Job drawing, mm, ordinate dimensions from the low corner. One solid piece. Coordinates: 2 decimals unless noted, no trailing zeros. Write each loop counter-clockwise with the first axis right and the second up, starting at its lowest first coordinate (ties: lowest second). Pieces come first, ordered by that corner, then holes. Notation, with made-up numbers: (-12, 26) -> (40, 26) arc R29 cw to (40, 52) -> close; hole circle Ø4 at (-24.75, 73.25). An arc over 180 degrees is marked (long way). Answer as a JSON object with one key per item and string values. Group by question number.
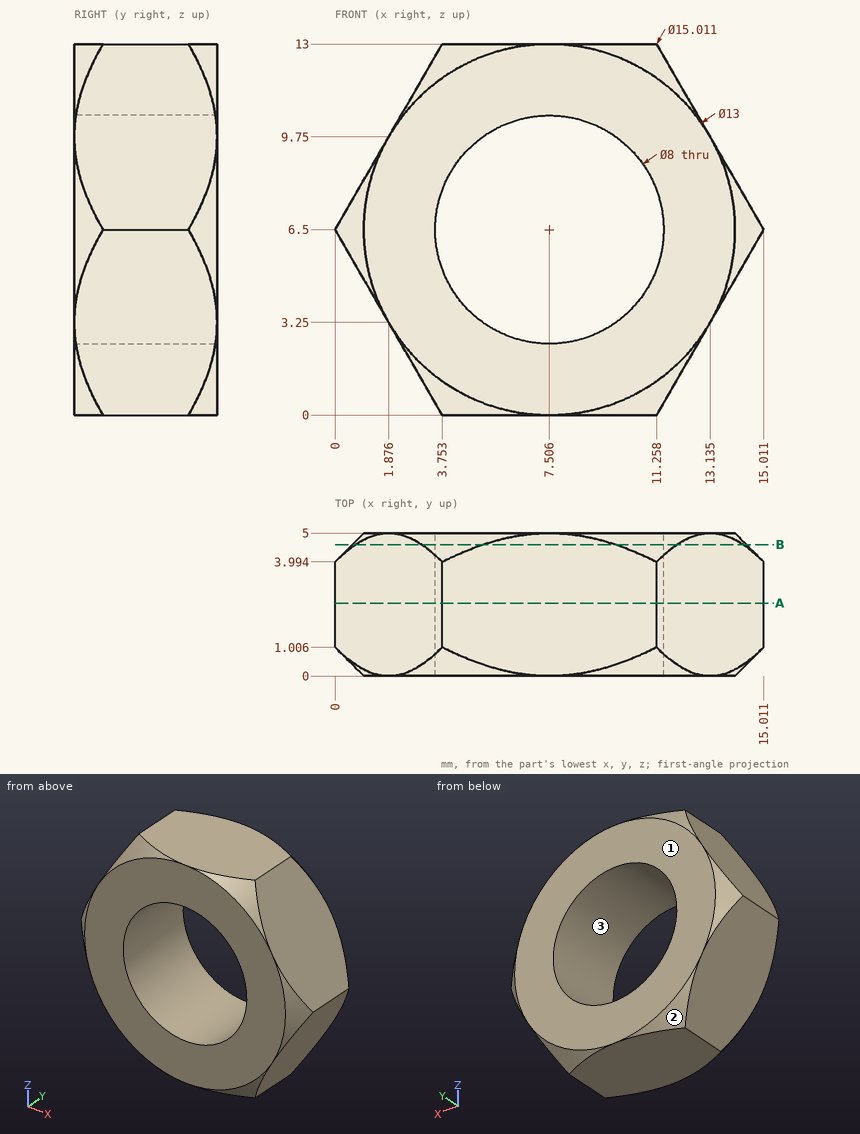
(1) Pin check, flat tip, straight feed: pin 1 (3 mm diameter, centred on y = 2, z = 3.5, fed in from -X) (1 decimal). Stop position of the tip, or through.
(2) Cut at A-A on y = 2.55. List the corners of the cut face in (x, z) (1 decimal).
(3) Pull direction X, two halves, no side cores. Call the marked faces 1, 2 and 3: released by +X, released by -X, zero draft, split by the parting line, or undercut.
(4) Wall check: probe 1 along Z at (x, y) = (6.25, 2.2); probe 2 along X at (y, z) = (1.5, 7.25) (1 decimal); probe 3 along Z at (x, y) = (7, 0.95). Give the ranges that are in metal, low to high.
(5) Cut at B-B on y = 4.6. List the corners of the cut face in (x, z) (1 decimal).
Results found:
{
 "1": {"pin 1": "stops at x = 0.9"},
 "2": {"outline": "(0, 6.5) -> (3.8, 0) -> (11.3, 0) -> (15, 6.5) -> (11.3, 13) -> (3.8, 13) -> close; hole circle Ø8 at (7.5, 6.5)"},
 "3": {"face 1": "zero draft", "face 2": "released by -X", "face 3": "undercut"},
 "4": {"probe 1": "z = 0 to 2.7, 10.3 to 13", "probe 2": "x = 0.4 to 3.6, 11.4 to 14.6", "probe 3": "z = 0 to 2.53, 10.47 to 13"},
 "5": {"outline": "(0.7, 5.3) -> (3, 1.2) arc R6.9 ccw to (5.2, 0) -> (9.8, 0) arc R6.9 ccw to (12, 1.2) -> (14.3, 5.3) arc R6.9 ccw to (14.3, 7.7) -> (12, 11.8) arc R6.9 ccw to (9.8, 13) -> (5.2, 13) arc R6.9 ccw to (3, 11.8) -> (0.7, 7.7) arc R6.9 ccw to start; hole circle Ø8 at (7.5, 6.5)"}
}
